```python
from build123d import *

# Parameters (mm, degrees)
F1_W     = 143.4
F1_H     = 143.4
F3_DEPTH = 0.6
F2_R     = 2.7
F4_DEPTH = 0.601
F5_R     = 4.6
F5_R_2   = 2.6
F6_DEPTH = 2


with BuildPart() as f3:
    # F1 (on Top) → F3 (new body)
    with BuildSketch(Plane.XY):
        Rectangle(F1_W, F1_H)
        with BuildLine():
            ThreePointArc((-69, 29.393877), (-53.033009, 53.033009), (-29.393877, 69))
            Line((-29.393877, 69), (29.393877, 69))
            ThreePointArc((29.393877, 69), (53.033009, 53.033009), (69, 29.393877))
            Line((69, 29.393877), (69, -29.393877))
            ThreePointArc((69, -29.393877), (53.033009, -53.033009), (29.393877, -69))
            Line((29.393877, -69), (-29.393877, -69))
            ThreePointArc((-29.393877, -69), (-53.033009, -53.033009), (-69, -29.393877))
            Line((-69, -29.393877), (-69, 29.393877))
        make_face(mode=Mode.SUBTRACT)
    extrude(amount=-F3_DEPTH)

    # F2 (on Top) → F4 (cut, through all)
    with BuildSketch(Plane.XY):
        with Locations((62.25, 62.25)):
            Circle(F2_R)
        with Locations((-62.25, 62.25)):
            Circle(F2_R)
        with Locations((-62.25, -62.25)):
            Circle(F2_R)
        with Locations((62.25, -62.25)):
            Circle(F2_R)
    extrude(amount=-F4_DEPTH, mode=Mode.SUBTRACT)

    # F5 (on Top) → F6 (join)
    with BuildSketch(Plane.XY):
        with Locations((-62.25, 62.25)):
            Circle(F5_R)
        with Locations((-62.25, 62.25)):
            Circle(F5_R_2, mode=Mode.SUBTRACT)
        with Locations((-62.25, -62.25)):
            Circle(F5_R)
        with Locations((-62.25, -62.25)):
            Circle(F5_R_2, mode=Mode.SUBTRACT)
        with Locations((62.25, -62.25)):
            Circle(F5_R)
        with Locations((62.25, -62.25)):
            Circle(F5_R_2, mode=Mode.SUBTRACT)
        with Locations((62.25, 62.25)):
            Circle(F5_R)
        with Locations((62.25, 62.25)):
            Circle(F5_R_2, mode=Mode.SUBTRACT)
    extrude(amount=F6_DEPTH)


solid = f3.part
```
Check sheet for the modelled part. Datum: model origin and axes. Units: mm. A direction names the side the tool comes from. Give positions to 0.01 mm unless a question says otherwise; leave off trailing zeros. Order: outer loops, then holes, each group sorted by start corner. A loop starts at its lowest first (then second) coordinate and runs counter-clockwise, first axis right, second up. Notation, with made-up numbers: M -18,-3.5 L 11,-3.5 A32 ccw 11,22.5 Z; hole C 76,55.25 d8. An arc over 180 degrees is marked long. Answer in a Markdown table with one row per item. Add a question column.
Q1. Gauge pin test, flat end, axial feed: pin 1 Ø3 at (x, y) = (62.25, -62.25) entering from +Z. Record the tip position at first contact, or that the pin passes through.
Q2. Sectioned sample at A-A, the plane z = 0.45. Record the boundary of the cut face in (x, y).
Q3. Access from +Z, -Z, +X, -X, +Y, -Y to the whole of each face (thin tool, end or side, straight path). Record for faces 3 (the flat face through (-60, 60, 2)), 4 (the cylindrical face through (-52.748, -53.316, -0.296)), 5 (the cylindrical face through (-66.846, -62.048, 0.986)).
Q4. Sectioned sample at C-C, the plane x = -62.25. Count the separate pieces of the cut face and the enclosed holes in it, and give its area (3 significant figures).
Q5. Release check for a two-part mould opening along X. For faces 1 (the flat face through (64.2, -64.2, 2)), 2 (the cylindrical face through (52.748, 53.316, -0.296)) record: released by +X, released by -X, zero draft, split by the parting line, or undercut.
Q6. Sectioned sample at B-B, the plane y = -26.5. Record the boundary of the cut face in (x, z).
Q7. Thickness scan on L1, parallel to Y at x = -62.25, z = 0.85; L2, parallel to Y at x = 22, z = -0.2; L3, parallel to Y at x = -62.25, z = -0.15. Record the ranges inside material, lowest first.
Verdict:
| question | item | result |
|---|---|---|
| 1 | pin 1 | through |
| 2 | outline | C -62.25,-62.25 d9.2; C -62.25,62.25 d9.2; C 62.25,-62.25 d9.2; C 62.25,62.25 d9.2; hole C -62.25,-62.25 d5.2; hole C -62.25,62.25 d5.2; hole C 62.25,-62.25 d5.2; hole C 62.25,62.25 d5.2 |
| 3 | face 3 | +Z, +X, -X, +Y, -Y |
| 3 | face 4 | +Z, -Z |
| 3 | face 5 | +Z |
| 4 | separate pieces | 4 |
| 4 | enclosed holes | 0 |
| 4 | area | 45.4 mm² |
| 5 | face 1 | zero draft |
| 5 | face 2 | undercut |
| 6 | outline | M -71.7,-0.6 L -69,-0.6 L -69,0 L -71.7,0 Z; M 69,-0.6 L 71.7,-0.6 L 71.7,0 L 69,0 Z |
| 7 | L1 | -66.85 to -64.85, -59.65 to -57.65, 57.65 to 59.65, 64.85 to 66.85 |
| 7 | L2 | -71.7 to -69, 69 to 71.7 |
| 7 | L3 | -71.7 to -64.95, -59.55 to -41.83, 41.83 to 59.55, 64.95 to 71.7 |
